from build123d import *

# Parameters (mm, degrees)
SKETCH1_W           = 121
SKETCH1_H           = 78
BOSS_EXTRUDE1_DEPTH = 13
SKETCH2_W           = 115
SKETCH2_H           = 70
CUT_EXTRUDE1_DEPTH  = 1
SKETCH4_W           = 20
SKETCH4_H           = 10
SKETCH4_W_2         = 11.824806853
SKETCH4_H_2         = 3.99711781
CUT_EXTRUDE2_DEPTH  = 2


with BuildPart() as part:
    # Sketch1 → Boss-Extrude1 (new body)
    with BuildSketch(Plane.XY):
        with Locations((60.5, 39)):
            Rectangle(SKETCH1_W, SKETCH1_H)
    extrude(amount=BOSS_EXTRUDE1_DEPTH)

    # Sketch2 → Cut-Extrude1 (cut)
    with BuildSketch(Plane(origin=(0, 0, 0), x_dir=(-1, 0, 0), z_dir=(0, 0, -1))):
        with Locations((-60.5, 38)):
            Rectangle(SKETCH2_W, SKETCH2_H)
    extrude(amount=-CUT_EXTRUDE1_DEPTH, mode=Mode.SUBTRACT)

    # Sketch4 → Cut-Extrude2 (cut)
    with BuildSketch(Plane(origin=(0, 78, 0), x_dir=(1, 0, 0), z_dir=(0, 1, 0))):
        with Locations((71, -6.5)):
            Rectangle(SKETCH4_W, SKETCH4_H)
        with Locations((49.790852201, -5.791105027)):
            Rectangle(SKETCH4_W_2, SKETCH4_H_2)
    extrude(amount=-CUT_EXTRUDE2_DEPTH, mode=Mode.SUBTRACT)


solid = part.part
Can you work these out from the model? Positions are in its coordinate system, mm. A direction names the side the tool comes from. Round coordinates to 2 decimals unless told otherwise and drop trailing zeros. Write each loop counter-clockwise with the first axis right and the second up, starting at its lowest first coordinate (ties: lowest second). Pieces come first, ordered by that corner, then holes. Notation, with made-up numbers: (-7, -36) - (23, -36) arc R32 cw to (23, 1) - close; hole circle Ø11 at (32, 18). An arc over 180 degrees is marked (long way). Write each question's results on one line, items separated by ' | '. Start each with the question number.
1) We'd pull the mould along X, two halves only. Please class faces 4 (the flat face through (71, 76, 6)), 5 (the flat face through (121, 38, 6)), 6 (the flat face through (60, 40, 13)), 7 (the flat face through (0, 38, 6)): released by +X, released by -X, zero draft, split by the parting line, or undercut.
2) Which directions (+Z, -Z, +X, -X, +Y, -Y) give clear straight access to the entire face, cutting with the end or side of a thin tool? Please do faces 1 (the flat face through (61, 38, 1)), 2 (the flat face through (50, 76, 6)), 3 (the flat face through (60, 0, 6)).
3) Suppose I cut it at A-A (x = 25.5). List the corners of the cut face in (y, z) for me.
4) Suppose I cut it at B-B (y = 69). List the corners of the cut face in (x, z) for me.
5) Please list where these lines run through material, in increasing order: line 1 (X direction, y = 36.5, z = 0.5); line 2 (Z direction, x = 81, y = 18.5); line 3 (Y direction, x = 78, z = 4.75).
6) Suppose I cut it at C-C (x = 46). List the corners of the cut face in (y, z) for me.
7) For pin 1 Ø5 at (x, z) = (68.5, 5) entering from +Y; pin 2 Ø4 at (x, y) = (63, 63.5) entering from -Z, each with a flat end and sliding along its axis, tell me the tip position at first contact or that it passes through.
Here are the results:
1) face 4: undercut | face 5: released by +X | face 6: zero draft | face 7: released by -X
2) face 1: -Z | face 2: +Y | face 3: +Z, -Z, +X, -X, -Y
3) outline: (0, 0) - (3, 0) - (3, 1) - (73, 1) - (73, 0) - (78, 0) - (78, 13) - (0, 13) - close
4) outline: (0, 0) - (3, 0) - (3, 1) - (118, 1) - (118, 0) - (121, 0) - (121, 13) - (0, 13) - close
5) line 1: x = 0 to 3, 118 to 121 | line 2: z = 1 to 13 | line 3: y = 0 to 76
6) outline: (0, 0) - (3, 0) - (3, 1) - (73, 1) - (73, 0) - (78, 0) - (78, 3.79) - (76, 3.79) - (76, 7.79) - (78, 7.79) - (78, 13) - (0, 13) - close
7) pin 1: stops at y = 76 | pin 2: stops at z = 1
